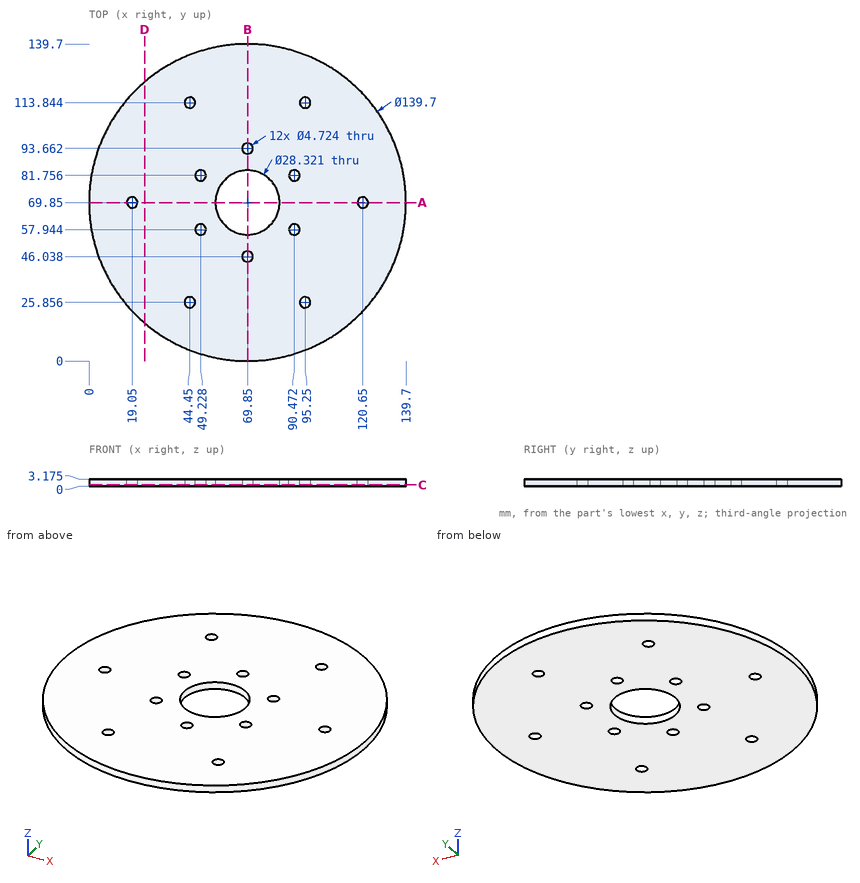
Study the drawing (mm; zero at the part's minimum x, y, z) and answer. Give positions to 0.01 mm unless a question says otherwise; leave off trailing zeros. Write each loop counter-clockwise with the first axis right and the second up, starting at its lowest first coordinate (ties: lowest second). Pieces come first, ordered by that corner, then holes. Notation, with made-up numbers: (42, 50.5) -> (54, 50.5) arc R15 ccw to (54, 68.5) -> close; hole circle Ø8 at (78.5, 49). An arc over 180 degrees is marked (long way). Write item = value, one per line. Start each with the question number.
1) The part is cut by section D-D, the plane x = 24.5. Determine the outline of the cut face in (y, z) (1 decimal).
2) The part is cut by section B-B, the plane x = 69.85. Determine the outline of the cut face in (y, z) (1 decimal).
3) Straight lines are drawn through the part: line 1 along Y through (x, z) = (50, 3) (1 decimal); line 2 along X through (y, z) = (70.5, 0.85) (1 decimal); line 3 along Y through (x, z) = (43, 1.3) (1 decimal). For each, find the intervals that lie inside material, in ascending order.
4) The part is cut by section A-A, the plane y = 69.85. Determine the outline of the cut face in (x, z) (1 decimal).
5) The part is cut by section C-C, the plane z = 0.55. Count the separate pieces of the cut face and the enclosed holes in it, and give its area (3 significant figures).
6) Each of these flat-tipped pins is pushed along its axis until it touches: pin 1 (4 mm diameter, centred on x = 120.65, y = 69.85, fed in from +Z); pin 2 (1.5 mm diameter, centred on x = 25, z = 2.5, fed in from -Y). Where does it stop, or does it pass through?
Solutions:
q1.outline = (16.7, 0) -> (123, 0) -> (123, 3.2) -> (16.7, 3.2) -> close
q2.outline = (0, 0) -> (43.7, 0) -> (43.7, 3.2) -> (0, 3.2) -> close; (48.4, 0) -> (55.7, 0) -> (55.7, 3.2) -> (48.4, 3.2) -> close; (84, 0) -> (91.3, 0) -> (91.3, 3.2) -> (84, 3.2) -> close; (96, 0) -> (139.7, 0) -> (139.7, 3.2) -> (96, 3.2) -> close
q3.line_1 = 2.9 to 55.7, 60.2 to 79.5, 84 to 136.8
q3.line_2 = 0 to 16.8, 21.3 to 55.7, 84 to 118.4, 122.9 to 139.7
q3.line_3 = 5.4 to 24, 27.7 to 112, 115.7 to 134.3
q4.outline = (0, 0) -> (16.7, 0) -> (16.7, 3.2) -> (0, 3.2) -> close; (21.4, 0) -> (55.7, 0) -> (55.7, 3.2) -> (21.4, 3.2) -> close; (84, 0) -> (118.3, 0) -> (118.3, 3.2) -> (84, 3.2) -> close; (123, 0) -> (139.7, 0) -> (139.7, 3.2) -> (123, 3.2) -> close
q5.separate_pieces = 1
q5.enclosed_holes = 13
q5.area = 14,500 mm²
q6.pin_1 = through
q6.pin_2 = 15.68
